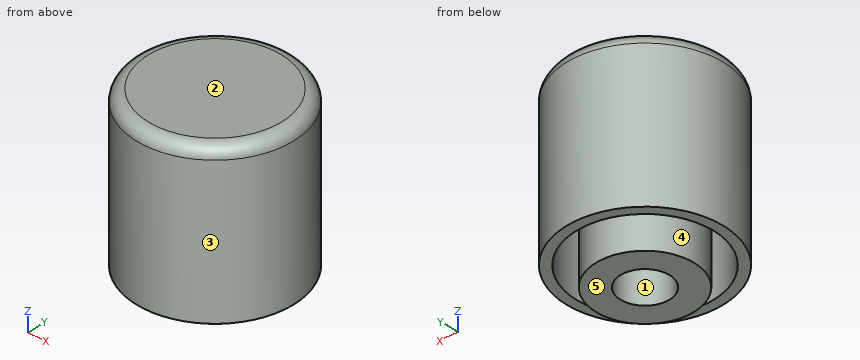
from build123d import *

# Parameters (mm, degrees)
F0_R     = 4
F1_DEPTH = 8
F2_R     = 0.6
F3_R     = 3.5
F4_DEPTH = 7
F5_R     = 2.5
F5_R_2   = 1.25
F6_DEPTH = 8


with BuildPart() as f1:
    # F0 (on Top) → F1 (new body)
    with BuildSketch(Plane.XY):
        Circle(F0_R)
    extrude(amount=F1_DEPTH)

    # F2
    f2_edges = [f1.edges().sort_by_distance(p)[0] for p in [
        (-4, 0, 8),
    ]]
    fillet(f2_edges, radius=F2_R)

    # F3 (on face) → F4 (cut)
    with BuildSketch(Plane(origin=(0, 0, 0), x_dir=(1, 0, 0), z_dir=(0, 0, -1))):
        Circle(F3_R)
    extrude(amount=-F4_DEPTH, mode=Mode.SUBTRACT)

    # F5 (on face) → F6 (join)
    with BuildSketch(Plane(origin=(0, 0, 7), x_dir=(1, 0, 0), z_dir=(0, 0, -1))):
        Circle(F5_R)
        Circle(F5_R_2, mode=Mode.SUBTRACT)
    extrude(amount=F6_DEPTH)


solid = f1.part
The listing builds one solid part. Answer for the finished solid, in the listing's coordinates (mm). Face numbers are marked on the shaded views. A direction names the side the tool comes from. Give positions to 0.01 mm unless a question says otherwise; leave off trailing zeros. Write each loop counter-clockwise with the first axis right and the second up, starting at its lowest first coordinate (ties: lowest second). Pieces come first, ordered by that corner, then holes.
1) Section D-D (z = 7.25) is taken. Write down the section's boundary in (x, y).
2) A tool of negligible diameter and unlimited length cuts with its end or side. For the marked faces 1 and 2, from which of +Z, -Z, +X, -X, +Y, -Y can it reach the whole face along a straight path? Write none if from no direction.
3) For a pull along Y with two mould halves and no side action, classify the marked faces 3, 4 and 5 as pulls with the +Y half, pulls with the -Y half, needs draft (parallel to the pull), parting line crosses it, or undercut.
4) Given P1, Ø4, axis at x = 2.5, z = 4.5, coming from the +Y side; P2, Ø1.5, axis at x = 1, z = 1.5, coming from the -Y side, each flat-ended and moving along its own axis, determine where each tip first touches the part or whether it passes through.
5) Section A-A (z = 4) is taken. Write down the section's boundary in (x, y).
6) Section B-B (y = 0) is taken. Write down the section's boundary in (x, z).
7) Find the intervals of material crossed by L1, parallel to Y at x = 0, z = 3.25; L2, parallel to X at y = 0.5, z = 6; L3, parallel to Y at x = 1, z = 0.75, in increasing order.
Response:
1. outline: circle Ø8 at (0, 0)
2. face 1: -Z
2. face 2: +Z, +X, -X, +Y, -Y
3. face 3: parting line crosses it
3. face 4: undercut
3. face 5: needs draft
4. P1: stops at y = 3.97
4. P2: stops at y = -3.99
5. outline: circle Ø8 at (0, 0); circle Ø5 at (0, 0); hole circle Ø7 at (0, 0); hole circle Ø2.5 at (0, 0)
6. outline: (-4, 0) - (-3.5, 0) - (-3.5, 7) - (-2.5, 7) - (-2.5, -1) - (-1.25, -1) - (-1.25, 7) - (1.25, 7) - (1.25, -1) - (2.5, -1) - (2.5, 7) - (3.5, 7) - (3.5, 0) - (4, 0) - (4, 7.4) arc R0.6 ccw to (3.4, 8) - (-3.4, 8) arc R0.6 ccw to (-4, 7.4) - close
7. L1: y = -4 to -3.5, -2.5 to -1.25, 1.25 to 2.5, 3.5 to 4
7. L2: x = -3.97 to -3.46, -2.45 to -1.15, 1.15 to 2.45, 3.46 to 3.97
7. L3: y = -3.87 to -3.35, -2.29 to -0.75, 0.75 to 2.29, 3.35 to 3.87
